Can you work these out from the model? Positions are in its coordinate system, mm. A direction names the side the tool comes from. Coordinates: 2 decimals unless noted, no trailing zeros. Loops run counter-clockwise (first coordinate to the right, second up) from the corner with the lowest first, then second, coordinate; pieces in that order, holes last. Notation, with made-up numbers: (44.25, 51.25) - (77.25, 51.25) arc R34 ccw to (77.25, 90.25) - close; hole circle Ø5 at (-15.75, 76.5). An arc over 180 degrees is marked (long way). Put each result on its own line as item: value. Start each with the question number.
from build123d import *

# Parameters (mm, degrees)
SKETCH1_R           = 50
BOSS_EXTRUDE1_DEPTH = 65
SKETCH2_R           = 4
BOSS_EXTRUDE2_DEPTH = 12
SKETCH3_R           = 5
CUT_EXTRUDE1_DEPTH  = 5
CIRPATTERN1_COUNT   = 8
SKETCH4_R           = 5
CUT_EXTRUDE2_DEPTH  = 5
CIRPATTERN2_COUNT   = 8


with BuildPart() as part:
    # Sketch1 → Boss-Extrude1 (new body, symmetric)
    with BuildSketch(Plane(origin=(0, 0, 0), x_dir=(0, 0, -1), z_dir=(1, 0, 0))):
        Circle(SKETCH1_R)
    extrude(amount=BOSS_EXTRUDE1_DEPTH, both=True)

    # Sketch2 → Boss-Extrude2 (add)
    with BuildSketch(Plane.ZY.offset(65)):
        Circle(SKETCH2_R)
    extrude(amount=BOSS_EXTRUDE2_DEPTH)

    # Sketch3 → Cut-Extrude1 (cut)
    with BuildSketch(Plane.ZY.offset(65)):
        with Locations((0, 35)):
            Circle(SKETCH3_R)
    cut_extrude1 = extrude(amount=-CUT_EXTRUDE1_DEPTH, mode=Mode.SUBTRACT)

    # CirPattern1: Cut-Extrude1 ×8 about axis
    cirpattern1_axis = Axis((0, 0, 0), (1, 0, 0))
    for i in range(1, CIRPATTERN1_COUNT):
        add(cut_extrude1.rotate(cirpattern1_axis, i * 360 / CIRPATTERN1_COUNT), mode=Mode.SUBTRACT)

    # Sketch4 → Cut-Extrude2 (cut)
    with BuildSketch(Plane(origin=(65, 0, 0), x_dir=(0, 0, -1), z_dir=(1, 0, 0))):
        with Locations((0, 35)):
            Circle(SKETCH4_R)
    cut_extrude2 = extrude(amount=-CUT_EXTRUDE2_DEPTH, mode=Mode.SUBTRACT)

    # CirPattern2: Cut-Extrude2 ×8 about axis
    cirpattern2_axis = Axis((0, 0, 0), (1, 0, 0))
    for i in range(1, CIRPATTERN2_COUNT):
        add(cut_extrude2.rotate(cirpattern2_axis, i * 360 / CIRPATTERN2_COUNT), mode=Mode.SUBTRACT)


solid = part.part
Q1. We'd pull the mould along Z, two halves only. Please class faces 3 (the cylindrical face through (-63, 39, 3)), 4 (the cylindrical face through (0.91, 15.02, -47.69)): released by +Z, released by -Z, zero draft, split by the parting line, or undercut.
Q2. Please list where these lines run through material, in increasing order: line 1 along X through (y, z) = (10, -44); line 2 along Y through (x, z) = (58, -0.5); line 3 along X through (y, z) = (-32.5, 3). Write a range as [from, to].
Q3. I want a section at B-B on y = -35. List the corners of the cut face in (x, z) for me.
Q4. I want a section at A-A on z = 0. List the corners of the cut face in (x, y) for me.
Q5. I want a section at C-C on x = -4. List the corners of the cut face in (y, z) for me.
Q6. On a 3-axis mill with a long thin cutter (end or side, diameter ignored), from which of +Z, -Z, +X, -X, +Y, -Y can I reach the whole of each face in a straight line? I mean faces 1 (the flat face through (60, -25, -25)), 2 (the flat face through (-60, -35, 0)). Say none if no direction works.
Q7. Will these pins go through, and if not, where does the flat tip stop? pin 1 (11 mm diameter, centred on y = -26.5, z = 23, fed in from -X); pin 2 (4 mm diameter, centred on x = -56.5, z = 10.5, fed in from -Y); pin 3 (1.5 mm diameter, centred on x = -53.5, y = -33.5, fed in from -Z).
Calculated:
1. face 3: undercut
1. face 4: split by the parting line
2. line 1: [-65, 65]
2. line 2: [-50, 50]
2. line 3: [-60, 60]
3. outline: (-65, -35.71) - (65, -35.71) - (65, -5) - (60, -5) - (60, 5) - (65, 5) - (65, 35.71) - (-65, 35.71) - (-65, 5) - (-60, 5) - (-60, -5) - (-65, -5) - close
4. outline: (-77, -4) - (-65, -4) - (-65, -30) - (-60, -30) - (-60, -40) - (-65, -40) - (-65, -50) - (65, -50) - (65, -40) - (60, -40) - (60, -30) - (65, -30) - (65, 30) - (60, 30) - (60, 40) - (65, 40) - (65, 50) - (-65, 50) - (-65, 40) - (-60, 40) - (-60, 30) - (-65, 30) - (-65, 4) - (-77, 4) - close
5. outline: circle Ø100 at (0, 0)
6. face 1: +X
6. face 2: -X
7. pin 1: x = -65
7. pin 2: y = -49.27
7. pin 3: z = -37.78
